Design review of the part built by this model. Coordinates are the model's own, in mm. Face numbers are marked on the shaded views. A direction names the side the tool comes from. Coordinates: 2 decimals unless noted, no trailing zeros. Loops run counter-clockwise (first coordinate to the right, second up) from the corner with the lowest first, then second, coordinate; pieces in that order, holes last. Notation, with made-up numbers: (20.5, 1.5) -> (73.5, 1.5) arc R5 ccw to (73.5, 8.5) -> close; hole circle Ø8 at (57.25, 88.5). An arc over 180 degrees is marked (long way). Answer as a JSON object with one key per item and string values.
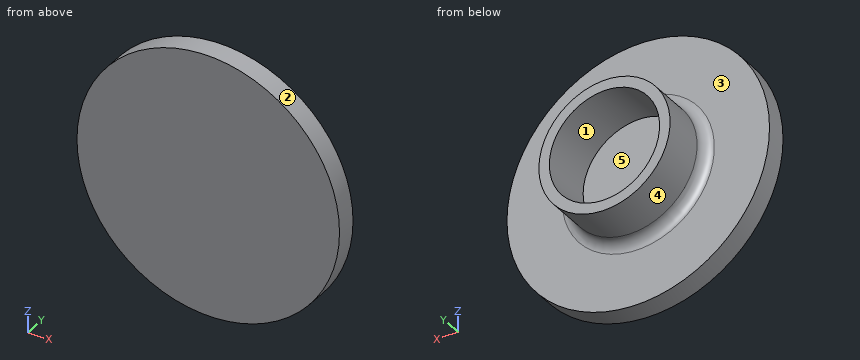
Autodesk Inventor part; units mm, degrees
ref_plane "YZ Plane" through (0, 0, 0) normal (1, 0, 0) x (0, 1, 0)
ref_plane "XZ Plane" through (0, 0, 0) normal (0, 1, 0) x (-1, 0, 0)
ref_plane "XY Plane" through (0, 0, 0) normal (0, 0, 1) x (1, 0, 0)
sketch "Sketch1" plane through (0, 0, 0) normal (0, 1, 0) x (-1, 0, 0)
  circle A0 centre (0, 0) radius 25
  dimension "d0" = 50
extrude "Extrusion1" add sketch "Sketch1" along normal blind 4
sketch "Sketch2" plane through (0, 4, 0) normal (0, 1, 0) x (1, 0, 0)
  circle A0 centre (0, 0) radius 12.5
  dimension "d3" = 25
extrude "Extrusion2" add sketch "Sketch2" along normal blind 10
sketch "Sketch3" plane through (0, 14, 0) normal (0, 1, 0) x (1, 0, 0)
  circle A0 centre (0, 0) radius 10.5
  dimension "d6" = 21
extrude "Extrusion3" cut sketch "Sketch3" against normal blind 10
fillet "Fillet1" radius 2 1 edges at (-12.5, 4, 0)
properties part number "Brida"
1) Add section A-A, the plane x = 0. Give the boundary of the cut face in (y, z), and give its area (3 significant figures).
Completed:
{"outline": "(0, -25) -> (4, -25) -> (4, -14.5) arc R2 cw to (6, -12.5) -> (14, -12.5) -> (14, -10.5) -> (4, -10.5) -> (4, 10.5) -> (14, 10.5) -> (14, 12.5) -> (6, 12.5) arc R2 cw to (4, 14.5) -> (4, 25) -> (0, 25) -> close", "area": "242 mm²"}
2) Add section D-D, the plane x = 21. Give the boundary of the cut face in (y, z).
Completed:
{"outline": "(0, -13.56) -> (4, -13.56) -> (4, 13.56) -> (0, 13.56) -> close"}
3) For the marked faces 1 and 2, list the 3-axis set-ups (+Z, -Z, +X, -X, +Y, -Y) from which the entire face can be reached by the end or side of a thin tool; tool diameter is ignored.
Completed:
{"face 1": "+Y", "face 2": "+Y, -Y"}
4) Add section C-C, the plane z = 0. Give the boundary of the cut face in (x, y), and give its area (3 significant figures).
Completed:
{"outline": "(-25, 0) -> (25, 0) -> (25, 4) -> (14.5, 4) arc R2 cw to (12.5, 6) -> (12.5, 14) -> (10.5, 14) -> (10.5, 4) -> (-10.5, 4) -> (-10.5, 14) -> (-12.5, 14) -> (-12.5, 6) arc R2 cw to (-14.5, 4) -> (-25, 4) -> close", "area": "242 mm²"}
5) Add section B-B, the plane y = 8.5. Give the boundary of the cut face in (x, z).
Completed:
{"outline": "circle Ø25 at (0, 0); hole circle Ø21 at (0, 0)"}
6) Wall thickness on probe 1 along Z at (x, y) = (0, 12.25); probe 2 along Y at (x, z) = (12.5, 13.5): over which ranges is each line inside the solid? List them lowest first.
Completed:
{"probe 1": "-12.5 to -10.5, 10.5 to 12.5", "probe 2": "0 to 4"}
7) The part is to be moulded in two halves that separate along Z. For the marked faces 3, 4 and 5, say which applies: pulls with the +Z half, pulls with the -Z half, needs draft (parallel to the pull), parting line crosses it, or undercut.
Completed:
{"face 3": "needs draft", "face 4": "parting line crosses it", "face 5": "undercut"}
8) Clearance check with flat-ended pins moving along their axes: pin 1 Ø8 at (x, z) = (14, 19.5) entering from +Y; pin 2 Ø1 at (y, z) = (8, -4.5) entering from -X; pin 3 Ø1.5 at (y, z) = (2, -7) entering from -X. State where each tip first meets the part, or that it passes through.
Completed:
{"pin 1": "y = 4", "pin 2": "x = -11.84", "pin 3": "x = -24.21"}
